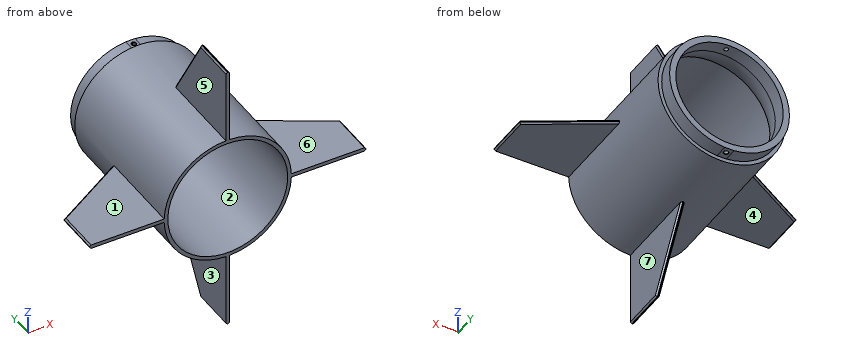
```python
from build123d import *

# Parameters (mm, degrees)
SKETCH1_W                    = 4.318
SKETCH1_H                    = 9.398
SKETCH1_W_2                  = 2.54
SKETCH1_H_2                  = 106.68
BOSS_EXTRUDE3_DEPTH          = 1.27
CHAMFER1_SIZE                = 1.016
CIRPATTERN6_COUNT            = 4
CHAMFER1_OF_CIRPATTERN6_SIZE = 1.016
CUT_EXTRUDE6_DEPTH           = 164.591183691
CUT_EXTRUDE6_DEPTH_BACK      = 164.591183691
CUT_EXTRUDE7_START           = -9.398
CUT_EXTRUDE7_DEPTH           = 188.317430146
CIRPATTERN7_COUNT            = 2
FILLET1_R                    = 0.254


with BuildPart() as part:
    # Sketch1 → Revolve1 (revolve)
    with BuildSketch(Plane.XY, mode=Mode.PRIVATE) as revolve1_sk:
        with BuildLine():
            Line((-37.0459, 83.23489827), (-41.3639, 83.23489827))
            Line((-41.3639, 83.23489827), (-41.3639, 69.51194771))
            ThreePointArc((-41.3639, 69.51194771), (-38.150873616, 76.041767935), (-37.0459, 83.23489827))
        make_face()
        with Locations((-39.2049, 87.93389827)):
            Rectangle(SKETCH1_W, SKETCH1_H)
        with Locations((-42.6339, 29.89489827)):
            Rectangle(SKETCH1_W_2, SKETCH1_H_2)
    revolve(revolve1_sk.sketch.rotate(Axis((0, 21.7161892, 0), (0, -1, 0)), 270), axis=Axis((0, 21.7161892, 0), (0, -1, 0)))

    # Sketch4 → Boss-Extrude3 (add, symmetric)
    with BuildSketch(Plane(origin=(0, 0, 0), x_dir=(0, 0, -1), z_dir=(1, 0, 0))):
        Polygon((43.805829154, -23.44510173), (43.805829154, 37.51489827), (95.344694503, 7.03489827), (95.344694503, -23.44510173), align=None)
    boss_extrude3 = extrude(amount=BOSS_EXTRUDE3_DEPTH, both=True)

    # Chamfer1
    chamfer1_edges = [part.edges().sort_by_distance(p)[0] for p in [
        (-1.27, -8.20510173, -95.344694503),
        (1.27, -8.20510173, -95.344694503),
        (-1.27, 22.251331497, -69.615111065),
        (1.27, 22.251331497, -69.615111065),
    ]]
    chamfer(chamfer1_edges, length=CHAMFER1_SIZE)

    # CirPattern6: Boss-Extrude3 ×4 about axis
    cirpattern6_axis = Axis((0, 0, 0), (0, 1, 0))
    for i in range(1, CIRPATTERN6_COUNT):
        add(boss_extrude3.rotate(cirpattern6_axis, i * 360 / CIRPATTERN6_COUNT))

    # Chamfer1 of CirPattern6
    chamfer1_of_cirpattern6_edges = [part.edges().sort_by_distance(p)[0] for p in [
        (-95.344694503, -8.20510173, 1.27),
        (-95.344694503, -8.20510173, -1.27),
        (-69.615111065, 22.251331497, 1.27),
        (-69.615111065, 22.251331497, -1.27),
        (1.27, -8.20510173, 95.344694503),
        (-1.27, -8.20510173, 95.344694503),
        (1.27, 22.251331497, 69.615111065),
        (-1.27, 22.251331497, 69.615111065),
        (95.344694503, -8.20510173, -1.27),
        (95.344694503, -8.20510173, 1.27),
        (69.615111065, 22.251331497, -1.27),
        (69.615111065, 22.251331497, 1.27),
    ]]
    chamfer(chamfer1_of_cirpattern6_edges, length=CHAMFER1_OF_CIRPATTERN6_SIZE)

    # Sketch6 → Cut-Extrude6 (cut, two sides: drawn at the far end of the back side and taken through both)
    with BuildSketch(Plane.XY.offset(-CUT_EXTRUDE6_DEPTH_BACK)):
        with BuildLine():
            Line((-0.771031735, 89.852901434), (0, 90.323685317))
            Line((0, 90.323685317), (0.771031735, 89.852901434))
            ThreePointArc((0.771031735, 89.852901434), (0, 87.110585317), (-0.771031735, 89.852901434))
        make_face()
    extrude(amount=CUT_EXTRUDE6_DEPTH + CUT_EXTRUDE6_DEPTH_BACK, mode=Mode.SUBTRACT)

    # Sketch7 → Cut-Extrude7 (cut)
    with BuildSketch(Plane(origin=(0, 92.63289827, 0), x_dir=(1, 0, 0), z_dir=(0, 1, 0)).offset(CUT_EXTRUDE7_START)):
        with BuildLine():
            ThreePointArc((0, 41.3639), (-1.601400576, 41.332889318), (-3.2004, 41.239903771))
            Line((-3.2004, 41.239903771), (3.2004, 41.239903771))
            ThreePointArc((3.2004, 41.239903771), (1.601400576, 41.332889318), (0, 41.3639))
        make_face()
    cut_extrude7 = extrude(amount=CUT_EXTRUDE7_DEPTH, mode=Mode.SUBTRACT)

    # CirPattern7: Cut-Extrude7 ×2 about axis
    cirpattern7_axis = Axis((0, 21.7161892, 0), (0, 1, 0))
    for i in range(1, CIRPATTERN7_COUNT):
        add(cut_extrude7.rotate(cirpattern7_axis, i * 360 / CIRPATTERN7_COUNT), mode=Mode.SUBTRACT)

    # Fillet1
    fillet1_edges = [part.edges().sort_by_distance(p)[0] for p in [
        (0.385515867, 90.088293375, -41.239903771),
        (0, 87.110585317, -41.239903771),
        (-0.385515867, 90.088293375, -41.239903771),
        (0, 87.110585317, 41.239903771),
        (-0.385515867, 90.088293375, 41.239903771),
        (0.385515867, 90.088293375, 41.239903771),
    ]]
    fillet(fillet1_edges, radius=FILLET1_R)


solid = part.part
```
The listing builds one solid part. Answer for the finished solid, in the listing's coordinates (mm). Face numbers are marked on the shaded views. A direction names the side the tool comes from. Give positions to 0.01 mm unless a question says otherwise; leave off trailing zeros. Loops run counter-clockwise (first coordinate to the right, second up) from the corner with the lowest first, then second, coordinate; pieces in that order, holes last. Notation, with made-up numbers: (-11, -25.5) - (48, -25.5) arc R21 cw to (48, -20.5) - close; hole circle Ø10 at (12.25, 79.5). An arc over 180 degrees is marked (long way). Return JSON: item names as keys, results as strings. Group by question number.
1. Given pin 1 Ø15 at (x, y) = (66, 0) entering from +Z; pin 2 Ø5 at (x, y) = (-1, 85.5) entering from +Z; pin 3 Ø1 at (y, z) = (-3, 51.5) entering from -X, each flat-ended and moving along its own axis, determine where each tip first touches the part or whether it passes through.
2. Find section D-D (y = 32.5). Write down the section's boundary in (x, z).
3. Which of the six approach directions +Z, -Z, +X, -X, +Y, -Y give full straight-line access (tool end or side, diameter ignored) to the marked faces 4, 5, 6 and 7?
4. Find section A-A (y = -6). Write down the section's boundary in (x, z), then the cut area to 3 significant figures.
5. Determine the mould class of the marked faces 1, 2 and 3 for opening direction X: pulls with the +X half, pulls with the -X half, needs draft (parallel to the pull), parting line crosses it, or undercut.
6. Find section C-C (z = -68.5). Write down the section's boundary in (x, y), then the cut area to 3 significant figures.
7. Straight lines are drawn through the part: line 1 (X direction, y = 87.5, z = 0); line 2 (X direction, y = 27, z = 2.5); line 3 (Z direction, x = -45.5, y = 25.5). For each, find the intervals that lie inside material, in ascending order. Write a range as [from, to].
8. Find section B-B (x = 59.5). Write down the section's boundary in (y, z), then the cut area to 3 significant figures.
Verdict:
{
 "1": {"pin 1": "stops at z = 1.27", "pin 2": "stops at z = 43.9", "pin 3": "stops at x = -1.27"},
 "2": {"outline": "(-52.29, -0.25) - (-50.29, -1.27) - (-43.89, -1.27) arc R43.9 ccw to (-1.27, -43.89) - (-1.27, -50.29) - (-0.25, -52.29) - (0.25, -52.29) - (1.27, -50.29) - (1.27, -43.89) arc R43.9 ccw to (43.89, -1.27) - (50.29, -1.27) - (52.29, -0.25) - (52.29, 0.25) - (50.29, 1.27) - (43.89, 1.27) arc R43.9 ccw to (1.27, 43.89) - (1.27, 50.29) - (0.25, 52.29) - (-0.25, 52.29) - (-1.27, 50.29) - (-1.27, 43.89) arc R43.9 ccw to (-43.89, 1.27) - (-50.29, 1.27) - (-52.29, 0.25) - close; hole circle Ø82.73 at (0, 0)"},
 "3": {"face 4": "-Z, -X, +Y, -Y", "face 5": "+Z, -X, +Y, -Y", "face 6": "+Z, +X, +Y, -Y", "face 7": "-Z, +X, +Y, -Y"},
 "4": {"outline": "(-95.34, -0.25) - (-94.33, -1.27) - (-43.89, -1.27) arc R43.9 ccw to (-1.27, -43.89) - (-1.27, -94.33) - (-0.25, -95.34) - (0.25, -95.34) - (1.27, -94.33) - (1.27, -43.89) arc R43.9 ccw to (43.89, -1.27) - (94.33, -1.27) - (95.34, -0.25) - (95.34, 0.25) - (94.33, 1.27) - (43.89, 1.27) arc R43.9 ccw to (1.27, 43.89) - (1.27, 94.33) - (0.25, 95.34) - (-0.25, 95.34) - (-1.27, 94.33) - (-1.27, 43.89) arc R43.9 ccw to (-43.89, 1.27) - (-94.33, 1.27) - (-95.34, 0.25) - close; hole circle Ø82.73 at (0, 0)", "area": "1,200 mm^2"},
 "5": {"face 1": "needs draft", "face 2": "undercut", "face 3": "pulls with the -X half"},
 "6": {"outline": "(-1.27, -23.45) - (1.27, -23.45) - (1.27, 21.73) - (0.25, 22.91) - (-0.25, 22.91) - (-1.27, 21.73) - close", "area": "117 mm^2"},
 "7": {"line 1": "x = [-41.36, -37.05], [37.05, 41.36]", "line 2": "x = [-43.83, -41.29], [41.29, 43.83]", "line 3": "z = [-1.27, 1.27]"},
 "8": {"outline": "(-23.45, -1.27) - (27.05, -1.27) - (28.23, -0.25) - (28.23, 0.25) - (27.05, 1.27) - (-23.45, 1.27) - close", "area": "130 mm^2"}
}
